Geometry: final body of the model. Coordinates: model frame, mm. Give positions to 0.01 mm unless a question says otherwise; leave off trailing zeros. Order: outer loops, then holes, each group sorted by start corner. A loop starts at its lowest first (then second) coordinate and runs counter-clockwise, first axis right, second up. Notation, with made-up numbers: (88.25, -7.75) - (131.25, -7.75) arc R22 ccw to (131.25, 19.25) - close; hole circle Ø2 at (26.5, 89). An arc over 180 degrees is marked (long way). Put each result on its own line as item: value. Start each with the question number.
1. Section B-B on x = 32. Return the cut outline in (y, z), plus the area to 3 significant figures.
2. First-contact query: P1, Ø7, axis at x = 15.1, z = -1.82, coming from the -Y side; P2, Ø2, axis at y = 2, z = -10, coming from the -X side. Flat tips, straight axial feed; report the tip coordinate or a pass-through.
3. Mould query, pull axis X, two halves, no side actions, for faces 1 (the flat face through (22, 2, 5.676)), 2 (the cylindrical face through (26.2, 1.8, -2.7)), 3 (the flat face through (47.235, 2, -24)). Classes: pulls with the +X half, pulls with the -X half, needs draft (parallel to the pull), parting line crosses it, or undercut.
4. Section C-C on y = 0.75. Return the cut outline in (x, z), plus the area to 3 significant figures.
5. Section D-D on z = -1.5. Return the cut outline in (x, y), plus the area to 3 significant figures.
6. Section A-A on z = -16.5. Return the cut outline in (x, y), plus the area to 3 significant figures.
7. Ray query, line 1 along X through (y, z) = (0.55, -2); line 2 along Z through (x, y) = (28.5, 0.7); line 3 along X through (y, z) = (3.35, -0.5). Return the intervals inside material, ascending. Write a range as from..to.
from build123d import *

# Parameters (mm, degrees)
BOSS_EXTRUDE1_DEPTH = 3.5
SKETCH2_R           = 4
CUT_EXTRUDE1_DEPTH  = 3.5


with BuildPart() as part:
    # Sketch1 → Boss-Extrude1 (new body)
    with BuildSketch(Plane(origin=(0, 0, 0), x_dir=(1, 0, 0), z_dir=(0, 1, 0))):
        Polygon((-2.765266864, -5.675626657), (47.234733136, -5.675626657), (47.234733136, 54.324373343), align=None)
    extrude(amount=BOSS_EXTRUDE1_DEPTH)

    # Sketch2 → Cut-Extrude1 (cut)
    with BuildSketch(Plane(origin=(0, 3.5, 0), x_dir=(1, 0, 0), z_dir=(0, 1, 0))):
        with Locations(Location((30.101973136, 1.824373343, 0), (0, 0, 270))):
            Circle(SKETCH2_R)
        with Locations(Location((15.101973136, 1.824373343, 0), (0, 0, 270))):
            Circle(SKETCH2_R)
        with Locations(Location((30.101973136, 16.824373343, 0), (0, 0, 270))):
            Circle(SKETCH2_R)
    extrude(amount=-CUT_EXTRUDE1_DEPTH, mode=Mode.SUBTRACT)


solid = part.part
Resolved:
1. outline: (0, -36.04) - (3.5, -36.04) - (3.5, -20.35) - (0, -20.35) - close; (0, -13.3) - (3.5, -13.3) - (3.5, -5.35) - (0, -5.35) - close; (0, 1.7) - (3.5, 1.7) - (3.5, 5.68) - (0, 5.68) - close
1. area: 96.7 mm^2
2. P1: through
2. P2: x = 9.46
3. face 1: needs draft
3. face 2: undercut
3. face 3: pulls with the +X half
4. outline: (-2.77, 5.68) - (47.23, -54.32) - (47.23, 5.68) - close; hole circle Ø8 at (15.1, -1.82); hole circle Ø8 at (30.1, -16.82); hole circle Ø8 at (30.1, -1.82)
4. area: 1,350 mm^2
5. outline: (3.21, 0) - (11.12, 0) - (11.12, 3.5) - (3.21, 3.5) - close; (19.09, 0) - (26.12, 0) - (26.12, 3.5) - (19.09, 3.5) - close; (34.09, 0) - (47.23, 0) - (47.23, 3.5) - (34.09, 3.5) - close
5. area: 98.3 mm^2
6. outline: (15.71, 0) - (26.12, 0) - (26.12, 3.5) - (15.71, 3.5) - close; (34.09, 0) - (47.23, 0) - (47.23, 3.5) - (34.09, 3.5) - close
6. area: 82.4 mm^2
7. line 1: 3.63..11.11, 19.1..26.11, 34.1..47.23
7. line 2: -31.84..-20.49, -13.16..-5.49, 1.84..5.68
7. line 3: 2.38..11.33, 18.88..26.33, 33.88..47.23
